```python
from build123d import *

# Parameters (mm, degrees)
F1_DEPTH = 25


with BuildPart() as f1:
    # F0 (on Top) → F1 (new body)
    with BuildSketch(Plane.XY):
        with BuildLine():
            ThreePointArc((-49.715382543, -55.6013963989), (-6.8009476536, -66.9407953487), (37.5171722726, -64.4639149259))
            ThreePointArc((37.5171722726, -64.4639149259), (61.5628712195, -27.1539289627), (72.9022701693, 15.7605059268))
            ThreePointArc((72.9022701693, 15.7605059268), (44.8488945123, 50.1587443216), (7.5389085491, 74.2044432685))
            ThreePointArc((7.5389085491, 74.2044432685), (-33.844730053, 58.1537377864), (-68.2429684479, 30.1003621294))
            ThreePointArc((-68.2429684479, 30.1003621294), (-65.7660880251, -14.2177577968), (-49.715382543, -55.6013963989))
        make_face()
    extrude(amount=F1_DEPTH)


solid = f1.part
```
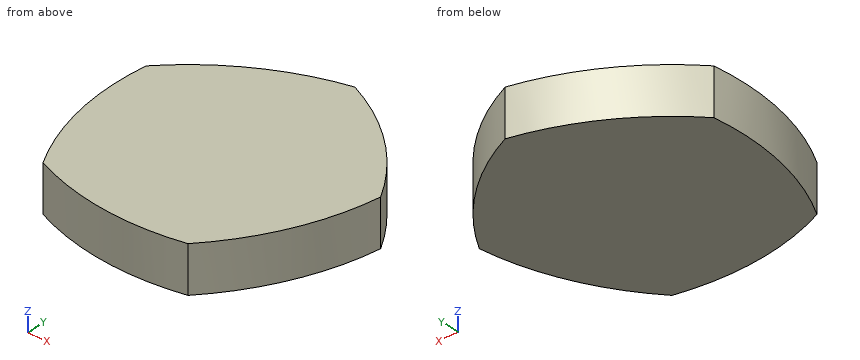
Geometry check sheet. Reference: the model listing, model coordinates, mm. Coordinates: 2 decimals unless noted, no trailing zeros. Order: outer loops, then holes, each group sorted by start corner. A loop starts at its lowest first (then second) coordinate and runs counter-clockwise, first axis right, second up. Notation, with made-up numbers: (38.5, 44) - (54.5, 44) arc R10 ccw to (54.5, 51) - close; hole circle Ø1 at (-22, 26). An arc over 180 degrees is marked (long way). Use one line per item in the form item = value.
1. Section check C-C (y = 56). Record the boundary of the cut face in (x, z).
Here are the results:
outline = (-37.42, 0) - (37.88, 0) - (37.88, 25) - (-37.42, 25) - close
2. Section check B-B (x = 27). Record the boundary of the cut face in (y, z).
Here are the results:
outline = (-66.33, 0) - (63.74, 0) - (63.74, 25) - (-66.33, 25) - close
3. Gauge pin test, flat ends, axial feed: pin 1 (2 mm diameter, centred on x = -44, z = 14.5, fed in from -Y); pin 2 (2 mm diameter, centred on x = 51.5, z = 14.5, fed in from +Y). Record the tip position at first contact, or that the pin passes through.
Here are the results:
pin_1 = -58.36
pin_2 = 44.82
4. Section check A-A (z = 10). Record the boundary of the cut face in (x, y).
Here are the results:
outline = (-68.24, 30.1) arc R141.87 ccw to (-49.72, -55.6) arc R141.87 ccw to (37.52, -64.46) arc R141.87 ccw to (72.9, 15.76) arc R141.87 ccw to (7.54, 74.2) arc R141.87 ccw to start
5. Scan lines: line 1 (X direction, y = -25.5, z = 14.5); line 2 (X direction, y = -45.5, z = 15.75); line 3 (Y direction, x = 46, z = 7). Record each from-to range of solid material in increasing order.
Here are the results:
line_1 = -62.84 to 62.28
line_2 = -55.06 to 51.81
line_3 = -54.02 to 49.12
